Autodesk Inventor part; units mm, degrees
ref_plane "YZ Plane" through (0, 0, 0) normal (1, 0, 0) x (0, 1, 0)
ref_plane "XZ Plane" through (0, 0, 0) normal (0, 1, 0) x (-1, 0, 0)
ref_plane "XY Plane" through (0, 0, 0) normal (0, 0, 1) x (1, 0, 0)
sketch "Skizze1" plane through (0, 0, 0) normal (0, 0, 1) x (1, 0, 0)
  line L0 (0, 0) -> (30, 0)
  line L1 (30, 0) -> (30, -2)
  line L2 (30, -2) -> (0, -2)
  line L3 (0, -2) -> (0, 0)
  line L4 (7.5, -2) -> (9.5, -2)
  line L5 (9.5, -2) -> (9.5, -22)
  line L6 (9.5, -22) -> (7.5, -22)
  line L7 (7.5, -22) -> (7.5, -2)
  line L8 (9.5, -22) -> (20.5, -22)
  line L9 (20.5, -22) -> (20.5, -20)
  line L10 (20.5, -20) -> (9.5, -20)
  line L11 (9.5, -20) -> (9.5, -22)
  line L12 (20.5, -22) -> (22.5, -22)
  line L13 (22.5, -22) -> (22.5, -2)
  line L14 (22.5, -2) -> (20.5, -2)
  line L15 (20.5, -2) -> (20.5, -22)
  line L16 (15, -20) -> (15, -2) construction
  point P0 (20.5, -2)
  point P1 (9.5, -2)
  dimension "d0" = 30
  dimension "d1" = 2
  dimension "d2" = 2
  dimension "d3" = 20
  dimension "d4" = 11
  dimension "d5" = 2
  dimension "d6" = 2
  dimension "d7" = 7.5
  dimension "d8" = 20.5
  dimension "d9" = 20
  dimension "d12" = 7.5
extrude "Extrusion1" add sketch "Skizze1" along normal blind 1000 contours L0 L1 L2 L3 | L2 L5 L6 L7 | L13 L12 L9 L15 L2 | L10 L9 L8 L5
sketch "Skizze2" plane through (22.5, -22, 0) normal (0, -1, 0) x (1, 0, 0)
  line L0 (7.5, 0) -> (7.5, 1000)
  line L1 (-26.5, 3) -> (11.5, 3)
  line L2 (11.5, 3) -> (11.5, 27)
  line L3 (-22.5, 0) -> (-22.5, 1000)
  line L4 (-26.5, 3) -> (-26.5, 27)
  line L5 (-26.5, 27) -> (11.5, 27)
  line L6 (-15, 0) -> (0, 0)
  line L7 (-26.5, 997) -> (11.5, 997)
  line L8 (11.5, 997) -> (11.5, 973)
  line L9 (11.5, 973) -> (-26.5, 973)
  line L10 (-26.5, 973) -> (-26.5, 997)
  line L11 (-15, 1000) -> (0, 1000)
  line L12 (0, 0) -> (0, 1000)
  line L13 (-15, 0) -> (-15, 1000)
  line L14 (-13, 0) -> (-13, 1000)
  point P0 (7.5, 3)
  point P1 (7.5, 27)
  dimension "d13" = 24
  dimension "d21" = 4
  dimension "d22" = 4
  dimension "d24" = 24
  dimension "d25" = 4
  dimension "d26" = 4
  dimension "d46" = 3
  dimension "d47" = 3
extrude "Extrusion2" add sketch "Skizze2" along normal blind 2 contours L1 L12 L5 L0 | L0 L5 L2 L1 | L1 L14 L5 L12 | L9 L12 L7 L0 | L0 L7 L8 L9 | L1 L13 L5 L14 | L9 L14 L7 L12 | L1 L3 L5 L13 | L9 L13 L7 L14 | L1 L4 L5 L3 | L9 L3 L7 L13 | L9 L10 L7 L3
sketch "Skizze3" plane through (22.5, -24, 0) normal (0, -1, 0) x (1, 0, 0)
  line L0 (-21, 15) -> (6, 15)
  line L1 (-15, 997) -> (-15, 1000)
  line L2 (-15, 0) -> (-15, 1000)
  line L3 (0, 0) -> (0, 1000)
  line L4 (0, 0) -> (0, 3)
  line L5 (6, 985) -> (-21, 985)
  line L6 (0, 27) -> (0, 973)
  line L7 (0, 3) -> (0, 27)
  line L8 (-15, 0) -> (-15, 3)
  line L9 (-15, 27) -> (-15, 973)
  line L10 (0, 997) -> (0, 1000)
  line L11 (0, 973) -> (0, 997)
  line L12 (-15, 3) -> (-15, 27)
  line L13 (-15, 973) -> (-15, 997)
  dimension "d19" = 6
  dimension "d23" = 15
  dimension "d27" = 6
  dimension "d28" = 6
  dimension "d48" = 15
hole "Bohrung1" at (1.5, -24, 15) at (28.5, -24, 15) at (1.5, -24, 985) at (28.5, -24, 985) direction (0, 1, 0) diameter 5.5 depth 2
properties part number "TrägerUI" material "Aluminium 6061, Katze"
Build history of the part. All positions in model axes, mm. A direction names the side the tool comes from. Give positions to 0.01 mm unless a question says otherwise; leave off trailing zeros. Order: outer loops, then holes, each group sorted by start corner. A loop starts at its lowest first (then second) coordinate and runs counter-clockwise, first axis right, second up. Notation, with made-up numbers: M 25.25,26.25 L 64.25,26.25 A21 cw 64.25,58.25 Z; hole C 43.5,-4 d9. An arc over 180 degrees is marked long. Put each result on its own line as item: value.
Item 1: Flat gauge pins, fed straight in: pin 1 Ø0.6 at (x, y) = (19.5, -23) entering from -Z; pin 2 Ø1 at (x, y) = (18, -23) entering from +Z; pin 3 Ø4.5 at (x, z) = (28.5, 985) entering from -Y; pin 4 Ø6.5 at (x, z) = (1.5, 985) entering from +Y. Where does each tip first touch, or does it go through?
From the geometry:
pin 1: stops at z = 3
pin 2: stops at z = 997
pin 3: stops at y = -2
pin 4: stops at y = 0
Item 2: 3-axis set-ups, long thin cutter, end or side, ignore diameter. For faces 1 (the flat face through (20.5, -11, 493)), 2 (the flat face through (15, -24, 15)): which of +Z, -Z, +X, -X, +Y, -Y reach the whole face in a straight line?
From the geometry:
face 1: +Z, -Z
face 2: +Z, -Z, +X, -X, -Y
Item 3: Two-plate mould, pull along X, no slides. Class faces 3 (the flat face through (7.5, -12, 493)), 4 (the flat face through (9, -8, 1000)), 5 (the flat face through (9.5, -11, 493)): +X half, -X half, draft (parallel to the pull), parting line (faces both ways), or undercut.
From the geometry:
face 3: -X half
face 4: draft
face 5: undercut
Item 4: Slice it at B-B, the plane z = 833. Write the cut outline in (x, y).
From the geometry:
outline: M 0,-2 L 7.5,-2 L 7.5,-22 L 22.5,-22 L 22.5,-2 L 30,-2 L 30,0 L 0,0 Z; hole M 9.5,-20 L 20.5,-20 L 20.5,-2 L 9.5,-2 Z
Item 5: Probe line 1 (X direction, y = -23.15, z = 15); line 2 (Z direction, x = 1.5, y = -22.4); line 3 (Y direction, x = 14.5, z = 114.5). List the from-to ranges inside material, lowest first. Write a range as [from, to].
From the geometry:
line 1: x = [-4, -1.25], [4.25, 25.75], [31.25, 34]
line 2: z = [3, 12.25], [17.75, 27], [973, 982.25], [987.75, 997]
line 3: y = [-22, -20], [-2, 0]
Item 6: Slice it at A-A, the plane y = -8.5. Write the cut outline in (x, z), plus the area to 3 significant figures.
From the geometry:
outline: M 7.5,0 L 9.5,0 L 9.5,1000 L 7.5,1000 Z; M 20.5,0 L 22.5,0 L 22.5,1000 L 20.5,1000 Z
area: 4,000 mm2
